Check sheet for the modelled part. Datum: model origin and axes. Units: mm. A direction names the side the tool comes from. Give positions to 0.01 mm unless a question says otherwise; leave off trailing zeros. Order: outer loops, then holes, each group sorted by start corner. A loop starts at its lowest first (then second) coordinate and runs counter-clockwise, first axis right, second up. Notation, with made-up numbers: (50, 32) -> (99, 32) arc R10 ccw to (99, 40) -> close; hole circle Ø6 at (35.5, 50.5). An arc over 180 degrees is marked (long way). Write each question's results on one line, items separated by ' | '.
Autodesk Inventor part; units mm, degrees
ref_plane "YZ Plane" through (0, 0, 0) normal (1, 0, 0) x (0, 1, 0)
ref_plane "XZ Plane" through (0, 0, 0) normal (0, 1, 0) x (-1, 0, 0)
ref_plane "XY Plane" through (0, 0, 0) normal (0, 0, 1) x (1, 0, 0)
sketch "Sketch1" plane through (0, 0, 0) normal (0, 1, 0) x (-1, 0, 0)
  line L0 (-24.6998, -28.575) -> (24.6998, -28.575)
  line L1 (24.6998, 28.575) -> (-24.6998, 28.575)
  line L2 (-24.6998, 28.575) -> (-24.6998, -28.575)
  line L3 (-24.6998, -28.575) -> (24.6998, 28.575) construction
  line L4 (24.6998, -28.575) -> (-24.6998, 28.575) construction
  arc A0 (55.0184, 10.3359) -> (71.8794, 13.215) centre (63.1598, 13.4684) ccw
  line L5 (74.3603, 0) -> (-43.8805, 0)
  arc A1 (71.8794, -13.215) -> (55.0184, -10.3359) centre (63.1598, -13.4684) ccw
  line L6 (71.8794, 13.215) -> (76.9002, 13.215)
  line L7 (76.9002, 13.215) -> (76.9002, -13.215)
  line L8 (76.9002, -13.215) -> (71.8794, -13.215)
  arc A2 (55.0184, 10.3359) -> (24.6998, 28.575) centre (28.155, 0) ccw
  arc A3 (24.6998, -28.575) -> (55.0184, -10.3359) centre (28.155, 0) ccw
  point P0 (0, 0)
  dimension "d1" = 57.15
  dimension "d2" = 101.6
extrude "Extrusion1" add sketch "Sketch1" along normal blind 44.45
hole "Hole1" at (24.6998, 22.0232, -0.5107) direction (-1, 0, 0) diameter 3.175 depth 25.4 tip angle 118
sketch "Sketch2" plane through (0, 44.45, 0) normal (0, 1, 0) x (1, 0, 0)
  circle A0 centre (-25.4, 0) radius 25.4
  circle A1 centre (-25.4, 0) radius 22.225
  point P0 (0, 0)
  dimension "d14" = 50.8
  dimension "d15" = 25.4
  dimension "d18" = 44.45
extrude "Extrusion3" add sketch "Sketch2" along normal blind 2.54
extrude "Extrusion4" add sketch "Sketch2" along normal blind 1.27 contours A1
fillet "Fillet1" radius 1.27 1 edges at (-50.8, 46.99, 0)
properties part number "Durometer_Sensor"
1. Gauge pin test, flat ends, axial feed: pin 1 Ø2.5 at (x, y) = (-75, 14) entering from +Z (3 decimals); pin 2 Ø13.5 at (x, z) = (-17, 6) entering from +Y; pin 3 Ø5.5 at (x, y) = (-73.5, 20) entering from -Z (3 decimals). Record the tip position at first contact, or that the pin passes through.
Verdict:
pin 1: stops at z = 13.215 | pin 2: stops at y = 45.72 | pin 3: stops at z = -13.215
2. Material ranges on probe 1 along Y at (x, z) = (14, -23.5); probe 2 along Z at (x, y) = (4, 9) (3 decimals); probe 3 along Z at (x, y) = (20, 23) (3 decimals), recorded low to high. Write a range as from..to.
Verdict:
probe 1: y = 0..44.45 | probe 2: z = -28.575..28.575 | probe 3: z = -28.575..-1.762, 0.741..28.575
3. Access from +Z, -Z, +X, -X, +Y, -Y to the whole of each face (thin tool, end or side, straight path). Record for faces 1 (the cylindrical face through (11.82, 20.68, -1.36)), 2 (the flat face through (-74, 22, -13.215)), 3 (the flat face through (-26, 45.72, 0)).
Verdict:
face 1: +X | face 2: -Z, -X, +Y, -Y | face 3: +Y
4. Mould release check, pull along Z, two halves, no side actions. Record for faces 4 (the flat face through (-14, 0, 0)), 5 (the conical face through (-1.488, 21.754, -0.451)), 6 (the cylindrical face through (-64.463, 21.914, -4.843)): +Z half, -Z half, draft (parallel to the pull), parting line (faces both ways), or undercut.
Verdict:
face 4: draft | face 5: undercut | face 6: -Z half
5. Section check A-A on y = 15.5. Record the cut outline in (x, z) (3 decimals), then the cut area to 3 significant figures.
Verdict:
outline: (-76.9, -13.215) -> (-71.879, -13.215) arc R8.723 cw to (-55.018, -10.336) arc R28.783 ccw to (-24.7, -28.575) -> (24.7, -28.575) -> (24.7, 28.575) -> (-24.7, 28.575) arc R28.783 ccw to (-55.018, 10.336) arc R8.723 cw to (-71.879, 13.215) -> (-76.9, 13.215) -> close | area: 4,650 mm^2
